For this review, take the finished solid that the model builds, in its own axes (mm). Face numbers are marked on the shaded views. A direction names the side the tool comes from. Coordinates: 2 decimals unless noted, no trailing zeros. Write each loop counter-clockwise with the first axis right and the second up, starting at its lowest first coordinate (ties: lowest second). Pieces come first, ordered by that corner, then holes. Notation, with made-up numbers: M 72,-12.5 L 117,-12.5 A22 ccw 117,5.5 Z; hole C 21,-20.75 d2. An arc over 180 degrees is marked long. Return JSON: item names as keys, results as strings.
```python
from build123d import *

# Parameters (mm, degrees)
SKETCH1_R                = 1.5
BOSS_EXTRUDE1_DEPTH      = 5
BOSS_EXTRUDE2_DEPTH      = 11
SKETCH3_W                = 2
SKETCH3_H                = 3.5
BOSS_EXTRUDE3_DEPTH      = 4
F_3_0_3_DIAMETER_HOLE2_D = 3


with BuildPart() as part:
    # Sketch1 → Boss-Extrude1 (new body)
    with BuildSketch(Plane(origin=(0, 0, 0), x_dir=(1, 0, 0), z_dir=(0, 1, 0))):
        with BuildLine():
            Line((24, -7.5), (24, -3.8))
            ThreePointArc((24, -3.8), (27.8, 0), (24, 3.8))
            Line((24, 3.8), (24, 7.5))
            Line((24, 7.5), (0, 7.5))
            ThreePointArc((0, 7.5), (-7.5, 0), (0, -7.5))
            Line((0, -7.5), (24, -7.5))
        make_face()
        with Locations(Location((20, 0, 0), (0, 0, 270))):
            Circle(SKETCH1_R, mode=Mode.SUBTRACT)
        with Locations(Location((24, 0, 0), (0, 0, 270))):
            Circle(SKETCH1_R, mode=Mode.SUBTRACT)
        with Locations(Location((0, 0, 0), (0, 0, 270))):
            Circle(SKETCH1_R, mode=Mode.SUBTRACT)
    extrude(amount=BOSS_EXTRUDE1_DEPTH)

    # Sketch2 → Boss-Extrude2 (add)
    with BuildSketch(Plane(origin=(0, 5, 0), x_dir=(1, 0, 0), z_dir=(0, 1, 0))):
        Polygon((0, -7.5), (0, -3.5), (24.024712411, -3.5), (24, -7.5), align=None)
        Polygon((24.024712411, 3.5), (24, 7.5), (0, 7.5), (0, 3.5), align=None)
    extrude(amount=BOSS_EXTRUDE2_DEPTH)

    # Sketch3 → Boss-Extrude3 (add)
    with BuildSketch(Plane(origin=(0, 5, 0), x_dir=(1, 0, 0), z_dir=(0, 1, 0))):
        Polygon((10, 0), (8, 0), (8, -3.5), (12, -3.5), (12, 0), align=None)
        with Locations((11, 1.75)):
            Rectangle(SKETCH3_W, SKETCH3_H)
        with Locations((9, 1.75)):
            Rectangle(SKETCH3_W, SKETCH3_H)
    extrude(amount=BOSS_EXTRUDE3_DEPTH)

    # Ø3.0 (3) Diameter Hole2 (through all)
    with Locations(Plane.XY.offset(7.5)):
        with Locations((19, 12.5), (5, 12.5)):
            Hole(F_3_0_3_DIAMETER_HOLE2_D / 2)


solid = part.part
```
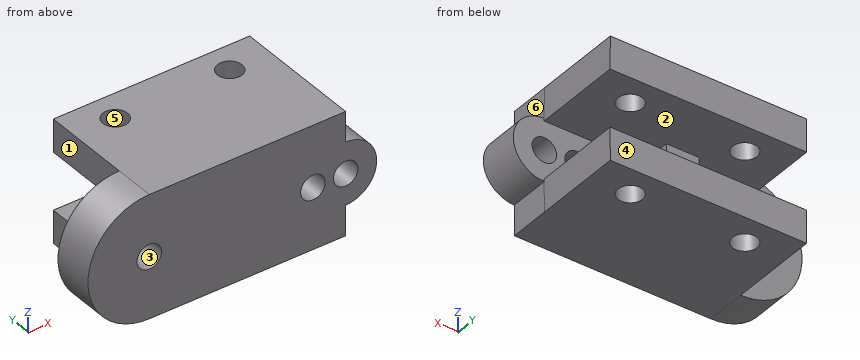
1. We need section C-C (x = 5). State the section outline as (y, z) points, plus the area to 3 significant figures.
Checks:
{"outline": "M 0,-7.5 L 11,-7.5 L 11,-3.5 L 5,-3.5 L 5,3.5 L 11,3.5 L 11,7.5 L 0,7.5 Z; M 14,-7.5 L 16,-7.5 L 16,-3.5 L 14,-3.5 Z; M 14,3.5 L 16,3.5 L 16,7.5 L 14,7.5 Z", "area": "139 mm2"}
2. Wall thickness on L1, parallel to X at y = 2, z = 0; L2, parallel to Y at x = 19, z = -6.5; L3, parallel to Z at x = 8, y = 14.5: over which ranges is each line inside the solid? List them lowest first. Write a range as from..to.
Checks:
{"L1": "-7.5..-1.5, 1.5..18.5, 21.5..22.5, 25.5..27.8", "L2": "0..11, 14..16", "L3": "-7.5..-3.5, 3.5..7.5"}
3. We need section D-D (x = 19). State the section outline as (y, z) points.
Checks:
{"outline": "M 0,-7.5 L 11,-7.5 L 11,-3.5 L 5,-3.5 L 5,-1.12 L 0,-1.12 Z; M 0,1.12 L 5,1.12 L 5,3.5 L 11,3.5 L 11,7.5 L 0,7.5 Z; M 14,-7.5 L 16,-7.5 L 16,-3.5 L 14,-3.5 Z; M 14,3.5 L 16,3.5 L 16,7.5 L 14,7.5 Z"}
4. Draft analysis for pull direction Y (two halves, no side actions). For the marked faces 4, 5 and 6, state which applies: +Y half, -Y half, draft (parallel to the pull), parting line (faces both ways), or undercut.
Checks:
{"face 4": "+Y half", "face 5": "undercut", "face 6": "draft"}
5. For the marked faces 1, 2 and 3, list the 3-axis set-ups (+Z, -Z, +X, -X, +Y, -Y) from which the entire face can be reached by the end or side of a thin tool; tool diameter is ignored.
Checks:
{"face 1": "+Z, -Z, -X, +Y", "face 2": "+Y", "face 3": "+Y, -Y"}
6. We need section B-B (z = 0). State the section outline as (x, y) points.
Checks:
{"outline": "M -7.5,0 L -1.5,0 L -1.5,5 L -7.5,5 Z; M 1.5,0 L 18.5,0 L 18.5,5 L 12,5 L 12,9 L 8,9 L 8,5 L 1.5,5 Z; M 21.5,0 L 22.5,0 L 22.5,5 L 21.5,5 Z; M 25.5,0 L 27.8,0 L 27.8,5 L 25.5,5 Z"}
7. Clearance check with flat-ended pins moving along their axes: pin 1 Ø1.8 at (y, z) = (3.5, 5) entering from +X; pin 2 Ø4 at (y, z) = (8, -0.5) entering from +X; pin 3 Ø6 at (y, z) = (3, 4.5) entering from -X. State where each tip first meets the part, or that it passes through.
Checks:
{"pin 1": "x = 24", "pin 2": "x = 12", "pin 3": "x = -7.35"}
8. We need section A-A (y = 14.75). State the section outline as (x, z) points, plus the area to 3 significant figures.
Checks:
{"outline": "M 0,-7.5 L 24,-7.5 L 24.02,-3.5 L 0,-3.5 Z; M 0,3.5 L 24.02,3.5 L 24,7.5 L 0,7.5 Z", "area": "192 mm2"}
